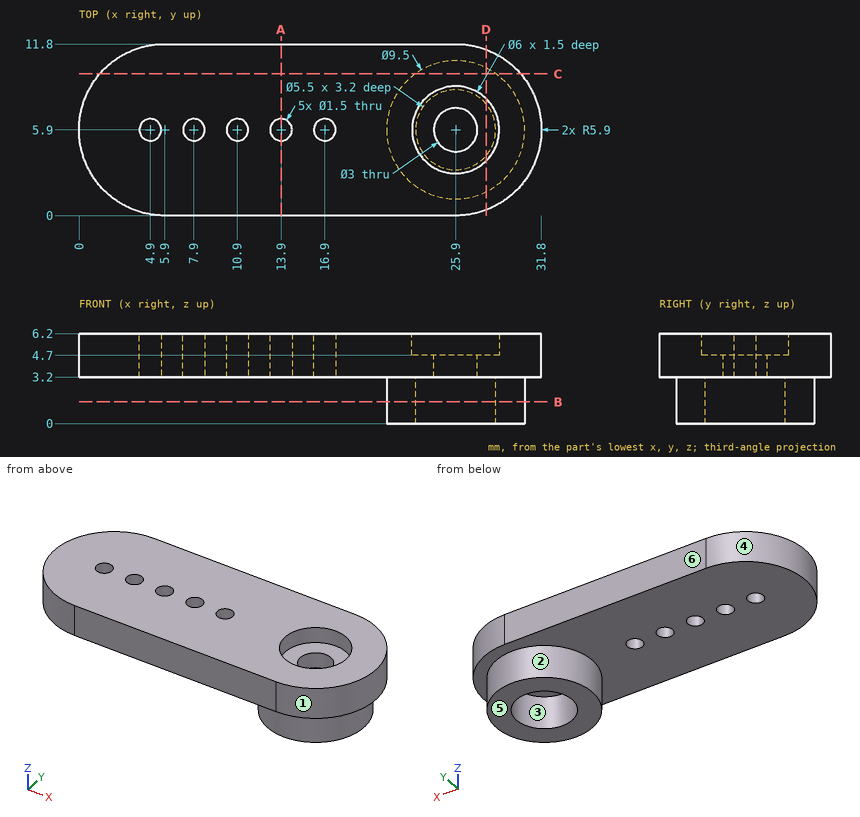
Part print with two shaded views. Sizes in mm from the minimum x, y, z corner. A direction names the side the tool comes from. Round coordinates to 2 decimals unless told otherwise and drop trailing zeros. Order: outer loops, then holes, each group sorted by start corner. A loop starts at its lowest first (then second) coordinate and runs counter-clockwise, first axis right, second up.
(1) Pull direction Y, two halves, no side cores. Call the marked faces 3, 4, 5 and 6: released by +Y, released by -Y, zero draft, split by the parting line, or undercut.
(2) Drill centre lines: line 1 (Y direction, x = 25.9, z = 5.4); line 2 (Y direction, x = 7.9, z = 5.2); line 3 (Z direction, x = 5, y = 1.75). Where is each one in solid material? Low to high.
(3) Band-saw the part on A-A (x = 13.9). List the corners of the cut face in (y, z).
(4) Band-saw the part on C-C (y = 9.75). List the corners of the cut face in (x, z).
(5) 3-axis set-ups, long thin cutter, end or side, ignore diameter. For the marked faces 1 and 2: which of +Z, -Z, +X, -X, +Y, -Y reach the whole face in a straight line?
(6) Pin check, flat tips, straight feed: pin 1 (2.5 mm diameter, centred on x = 16.9, y = 5.9, fed in from -Z); pin 2 (1 mm diameter, centred on x = 17, z = 2.5, fed in from -Y); pin 3 (5 mm diameter, centred on x = 25, y = 6.5, fed in from +Z); pin 4 (5.5 mm diameter, centred on x = 25.9, y = 5.9, fed in from +Z). Stop position of each tip, or through.
(7) Band-saw the part on D-D (x = 28). List the corners of the cut face in (y, z), then the cut area to 3 significant figures.
(8) Band-saw the part on B-B (z = 1.5). List the corners of the cut face in (x, y), then the cut area to 3 significant figures.
Verdict:
1. face 3: undercut
1. face 4: split by the parting line
1. face 5: zero draft
1. face 6: released by +Y
2. line 1: y = 0 to 2.9, 8.9 to 11.8
2. line 2: y = 0 to 5.15, 6.65 to 11.8
2. line 3: z = 3.2 to 6.2
3. outline: (0, 3.2) - (5.15, 3.2) - (5.15, 6.2) - (0, 6.2) - close; (6.65, 3.2) - (11.8, 3.2) - (11.8, 6.2) - (6.65, 6.2) - close
4. outline: (1.43, 3.2) - (23.12, 3.2) - (23.12, 0) - (28.68, 0) - (28.68, 3.2) - (30.37, 3.2) - (30.37, 6.2) - (1.43, 6.2) - close
5. face 1: +Z, -Z, +X
5. face 2: -Z
6. pin 1: stops at z = 3.2
6. pin 2: passes through
6. pin 3: stops at z = 6.2
6. pin 4: stops at z = 4.7
7. outline: (0.39, 3.2) - (1.64, 3.2) - (1.64, 0) - (4.12, 0) - (4.12, 3.2) - (7.68, 3.2) - (7.68, 0) - (10.16, 0) - (10.16, 3.2) - (11.41, 3.2) - (11.41, 6.2) - (8.04, 6.2) - (8.04, 4.7) - (3.76, 4.7) - (3.76, 6.2) - (0.39, 6.2) - close
7. area: 42.6 mm2
8. outline: circle Ø9.5 at (25.9, 5.9); hole circle Ø5.5 at (25.9, 5.9)
8. area: 47.1 mm2
